```python
from build123d import *

# Parameters (mm, degrees)
CROQUIS1_W              = 45
CROQUIS1_H              = 45
CROQUIS1_R              = 16
SALIENTE_EXTRUIR1_DEPTH = 15
CROQUIS2_R              = 1.5
CORTAR_EXTRUIR1_DEPTH   = 15
SALIENTE_EXTRUIR2_DEPTH = 15


with BuildPart() as part:
    # Croquis1 → Saliente-Extruir1 (new body)
    with BuildSketch(Plane.XY):
        Rectangle(CROQUIS1_W, CROQUIS1_H)
        Circle(CROQUIS1_R, mode=Mode.SUBTRACT)
    extrude(amount=SALIENTE_EXTRUIR1_DEPTH)

    # Croquis2 → Cortar-Extruir1 (cut)
    with BuildSketch(Plane.XY.offset(15)):
        with Locations((-17.5, 17.5)):
            Circle(CROQUIS2_R)
        with Locations((17.5, -17.5)):
            Circle(CROQUIS2_R)
        with Locations((-17.5, -17.5)):
            Circle(CROQUIS2_R)
        with Locations((17.5, 17.5)):
            Circle(CROQUIS2_R)
    extrude(amount=-CORTAR_EXTRUIR1_DEPTH, mode=Mode.SUBTRACT)

    # Croquis3 → Saliente-Extruir2 (add)
    with BuildSketch(Plane(origin=(22.5, 0, 0), x_dir=(0, 0, -1), z_dir=(1, 0, 0))):
        Polygon((-2, 0), (-2, 5), (0, 5), (0, -5), (-2, -5), align=None)
    saliente_extruir2 = extrude(amount=SALIENTE_EXTRUIR2_DEPTH)

    # Simetría1: Saliente-Extruir2 across plane
    add(saliente_extruir2.mirror(Plane(origin=(0, 0, 0), x_dir=(0, 0, 1), z_dir=(1, 0, 0))))


solid = part.part
```
CAD build for the part. Positions are in the model's coordinates, mm. A direction names the side the tool comes from. Give positions to 0.01 mm unless a question says otherwise; leave off trailing zeros. Write each loop counter-clockwise with the first axis right and the second up, starting at its lowest first coordinate (ties: lowest second). Pieces come first, ordered by that corner, then holes. Notation, with made-up numbers: M 72,88 L 79,88 A26 ccw 79,125 Z; hole C -14,16 d7. An arc over 180 degrees is marked long. Return JSON: item names as keys, results as strings. Group by question number.
(1) Band-saw the part on D-D (x = 0). Give the cut face in (y, z).
(2) 3-axis set-ups, long thin cutter, end or side, ignore diameter. For faces 4 (the face through (-30, -5, 1)), 5 (the face through (30, 5, 1)), 6 (the face through (30, 0, 2)), 7 (the face through (-30, 0, 2)): which of +Z, -Z, +X, -X, +Y, -Y reach the whole face in a straight line?
(3) Drill centre lines: L1, parallel to Y at x = -17.5, z = 5.25; L2, parallel to Y at x = 18.5, z = 8; L3, parallel to Y at x = 0, z = 6.5. Where is each one in solid material? Low to high. Write a range as [from, to].
(4) Flat gauge pins, fed straight in: pin 1 Ø1.8 at (x, y) = (-17.5, -17.5) entering from -Z; pin 2 Ø2 at (x, z) = (33, 1.5) entering from -Y; pin 3 Ø1.6 at (x, z) = (-29.5, 0.5) entering from +Y; pin 4 Ø8 at (x, y) = (33.5, -1.5) entering from +Z. Where does each tip first touch, or does it go through?
(5) Mould opens along Y. For faces 1 (the face through (0, -22.5, 7)), 2 (the face through (-22.5, 0, 7)), 3 (the face through (-18.61, 18.51, 7.6)) say: pulls with the +Y half, pulls with the -Y half, needs draft (parallel to the pull), parting line crosses it, or undercut.
(6) Band-saw the part on A-A (y = 17.5). Give the cut face in (x, z), and give its area (3 significant figures).
(7) Band-saw the part on B-B (z = 13.5). Give the cut face in (x, y).
Entries:
{
 "1": {"outline": "M -22.5,0 L -16,0 L -16,15 L -22.5,15 Z; M 16,0 L 22.5,0 L 22.5,15 L 16,15 Z"},
 "2": {"face 4": "+Z, -Z, -X, -Y", "face 5": "+Z, -Z, +X, +Y", "face 6": "+Z, +X, +Y, -Y", "face 7": "+Z, -X, +Y, -Y"},
 "3": {"L1": "y = [-22.5, -19], [-16, 16], [19, 22.5]", "L2": "y = [-22.5, -18.62], [-16.38, 16.38], [18.62, 22.5]", "L3": "y = [-22.5, -16], [16, 22.5]"},
 "4": {"pin 1": "passes through", "pin 2": "stops at y = -5", "pin 3": "stops at y = 5", "pin 4": "stops at z = 2"},
 "5": {"face 1": "pulls with the -Y half", "face 2": "needs draft", "face 3": "undercut"},
 "6": {"outline": "M -22.5,0 L -19,0 L -19,15 L -22.5,15 Z; M -16,0 L 16,0 L 16,15 L -16,15 Z; M 19,0 L 22.5,0 L 22.5,15 L 19,15 Z", "area": "585 mm^2"},
 "7": {"outline": "M -22.5,-22.5 L 22.5,-22.5 L 22.5,22.5 L -22.5,22.5 Z; hole C -17.5,-17.5 d3; hole C -17.5,17.5 d3; hole C 0,0 d32; hole C 17.5,-17.5 d3; hole C 17.5,17.5 d3"}
}
